Input: part model. Units: mm. Frame: model coordinates. Give positions to 0.01 mm unless a question says otherwise; leave off trailing zeros. Loops run counter-clockwise (first coordinate to the right, second up) from the corner with the lowest first, then second, coordinate; pieces in that order, holes last. Notation, with made-up numbers: (23.25, -26.75) -> (68.25, -26.75) arc R31 ccw to (68.25, 3.25) -> close; hole circle Ø3 at (27.5, 57). An arc over 180 degrees is marked (long way). One line per question, with ' | ' between items.
from build123d import *

# Parameters (mm, degrees)
F1_DEPTH = 527.05
F2_W     = 11.8364
F2_H     = 6.35
F3_DEPTH = 114.301


with BuildPart() as f1:
    # F0 (on Right) → F1 (new body)
    with BuildSketch(Plane.YZ):
        Polygon((0, 0), (-11.811, 0), (-11.811, -101.544328), (-11.811, -104.719328), (-11.811, -114.3), (0, -114.3), (0, -104.775), (-6.35, -104.775), (-6.35, -101.6), (0, -101.6), align=None)
    extrude(amount=-F1_DEPTH)

    # F2 (on Top) → F3 (cut, through all)
    with BuildSketch(Plane.XY):
        with Locations((-25.8318, -3.175)):
            Rectangle(F2_W, F2_H)
        with Locations((-501.2182, -3.175)):
            Rectangle(F2_W, F2_H)
    extrude(amount=-F3_DEPTH, mode=Mode.SUBTRACT)


solid = f1.part
1. Pull-direction query (X, two-part tool) for faces 1 (the flat face through (-265, -6.35, -103)), 2 (the flat face through (0, -6, -56)), 3 (the flat face through (-527.05, -6, -56)), 4 (the flat face through (-260, -6, -114.3)); classes: pulls with the +X half, pulls with the -X half, needs draft (parallel to the pull), parting line crosses it, or undercut.
Determined:
face 1: undercut | face 2: pulls with the +X half | face 3: pulls with the -X half | face 4: needs draft
2. Ray query, line 1 along X through (y, z) = (-2.5, -9.5); line 2 along Z through (x, y) = (-61, -1.75) (3 decimals). Return the intervals inside material, ascending. Write a range as from..to.
Determined:
line 1: x = -527.05..-507.14, -495.3..-31.75, -19.91..0 | line 2: z = -114.3..-104.775, -101.6..0
3. Section query A-A (y = -2.5). Output: boundary loops of the cut face in (x, z) (3 decimals), then the cut area to 3 significant figures.
Determined:
outline: (-527.05, -114.3) -> (-507.136, -114.3) -> (-507.136, -104.775) -> (-527.05, -104.775) -> close; (-527.05, -101.6) -> (-507.136, -101.6) -> (-507.136, 0) -> (-527.05, 0) -> close; (-495.3, -114.3) -> (-31.75, -114.3) -> (-31.75, -104.775) -> (-495.3, -104.775) -> close; (-495.3, -101.6) -> (-31.75, -101.6) -> (-31.75, 0) -> (-495.3, 0) -> close; (-19.914, -114.3) -> (0, -114.3) -> (0, -104.775) -> (-19.914, -104.775) -> close; (-19.914, -101.6) -> (0, -101.6) -> (0, 0) -> (-19.914, 0) -> close | area: 55,900 mm2
4. Section query B-B (z = -49). Output: boundary loops of the cut face in (x, y).
Determined:
outline: (-527.05, -11.81) -> (0, -11.81) -> (0, 0) -> (-19.91, 0) -> (-19.91, -6.35) -> (-31.75, -6.35) -> (-31.75, 0) -> (-495.3, 0) -> (-495.3, -6.35) -> (-507.14, -6.35) -> (-507.14, 0) -> (-527.05, 0) -> close
